```python
from build123d import *

# Parameters (mm, degrees)
TROU_TARAUD_M3X0_51_D     = 2.5
TROU_TARAUD_M3X0_51_DEPTH = 4
TROU_TARAUD_M3X0_51_TIP   = 0.751075774
CHANFREIN1_SIZE           = 0.5
CHANFREIN2_SIZE           = 1
CONG_1_R                  = 1
CHANFREIN3_SIZE           = 1
ESQUISSE4_W               = 15
ESQUISSE4_H               = 6
ENL_V_MAT_EXTRU_1_DEPTH   = 1


with BuildPart() as part:
    # Esquisse1 → Révolution1 (revolve)
    with BuildSketch(Plane.XY):
        Polygon((0, 0), (0, 3), (17, 3), (17, 10), (20, 10), (20, 16), (67, 16), (67, 0), align=None)
    revolve(axis=Axis((67, 0, 0), (-1, 0, 0)))

    # Trou taraudé M3x0.51
    with Locations(Plane.ZY.offset(-20)):
        with Locations((-13, 0), (0, 13), (13, 0), (0, -13)):
            Hole(TROU_TARAUD_M3X0_51_D / 2, depth=TROU_TARAUD_M3X0_51_DEPTH)
            with Locations((0, 0, -(TROU_TARAUD_M3X0_51_DEPTH + TROU_TARAUD_M3X0_51_TIP / 2))):  # 118° drill point
                Cone(0, TROU_TARAUD_M3X0_51_D / 2, TROU_TARAUD_M3X0_51_TIP, mode=Mode.SUBTRACT)

    # Chanfrein1
    chanfrein1_edges = [part.edges().sort_by_distance(p)[0] for p in [
        (67, -16, 0),
    ]]
    chamfer(chanfrein1_edges, length=CHANFREIN1_SIZE)

    # Chanfrein2
    chanfrein2_edges = [part.edges().sort_by_distance(p)[0] for p in [
        (20, -16, 0),
    ]]
    chamfer(chanfrein2_edges, length=CHANFREIN2_SIZE)

    # Congé1
    cong_1_edges = [part.edges().sort_by_distance(p)[0] for p in [
        (17, -10, 0),
    ]]
    fillet(cong_1_edges, radius=CONG_1_R)

    # Chanfrein3
    chanfrein3_edges = [part.edges().sort_by_distance(p)[0] for p in [
        (0, -3, 0),
    ]]
    chamfer(chanfrein3_edges, length=CHANFREIN3_SIZE)

    # Esquisse4 → Enlèv. mat.-Extru.1 (cut)
    with BuildSketch(Plane(origin=(0, 3, 0), x_dir=(1, 0, 0), z_dir=(0, 1, 0))):
        with Locations((7.5, 0)):
            Rectangle(ESQUISSE4_W, ESQUISSE4_H)
    extrude(amount=-ENL_V_MAT_EXTRU_1_DEPTH, mode=Mode.SUBTRACT)


solid = part.part
```
Source: CAD feature listing. Evaluate the final solid. Frame: model axes, mm. A direction names the side the tool comes from. Coordinates: 2 decimals unless noted, no trailing zeros. Write each loop counter-clockwise with the first axis right and the second up, starting at its lowest first coordinate (ties: lowest second). Pieces come first, ordered by that corner, then holes. Notation, with made-up numbers: (-33.75, -6.5) - (12.25, -6.5) arc R11 cw to (12.25, 12.5) - close; hole circle Ø6 at (71, 38.5). An arc over 180 degrees is marked (long way). Answer as a JSON object with one key per item and string values.
Q1. Set-up query: faces 1 (the flat face through (7, 2, 0)), 2 (the cylindrical face through (44.07, -3.47, 15.62)), 3 (the flat face through (17, 0, 4)). Return all of +Z, -Z, +X, -X, +Y, -Y with unobstructed straight access to the full face (end or side cutting, diameter ignored); none if empty.
Ans:
{"face 1": "+Z, -Z, -X, +Y", "face 2": "+X, -X", "face 3": "-X"}
Q2. Draft query along Z for faces 4 (the cylindrical face through (9, -3, 0)), 5 (the conical face through (24.62, 12.92, 0.2)), 6 (the flat face through (67, 0, 0)), 7 (the conical face through (24.621, -0.132, 12.828)). Return one class per face: released by +Z, released by -Z, zero draft, split by the parting line, or undercut.
Ans:
{"face 4": "split by the parting line", "face 5": "undercut", "face 6": "zero draft", "face 7": "undercut"}
Q3. Section query A-A, the plane x = 41. Output: boundary loops of the cut face in (y, z).
Ans:
{"outline": "circle Ø32 at (0, 0)"}
Q4. Material intervals for line 1 (Y direction, x = 23, z = 0); line 2 (X direction, y = -1, z = 5), sorted ascending. Write a range as [from, to].
Ans:
{"line 1": "y = [-16, -14.25], [-11.75, 11.75], [14.25, 16]", "line 2": "x = [17, 67]"}
Q5. First-contact query: pin 1 Ø1 at (x, z) = (10.5, -1.5) entering from -Y; pin 2 Ø4 at (y, z) = (0, -13) entering from -X; pin 3 Ø6 at (x, z) = (29, 7) entering from -Y; pin 4 Ø10 at (y, z) = (1, -5.5) entering from -X. Flat tips, straight axial feed; report the tip coordinate or a pass-through.
Ans:
{"pin 1": "stops at y = -2.83", "pin 2": "stops at x = 20", "pin 3": "stops at y = -15.49", "pin 4": "stops at x = 0"}
